The figure shows three views and two pictorial views of one solid part (mm, origin at its lowest corner). Answer the questions. A direction names the side the tool comes from. Give positions to 0.01 mm unless a question says otherwise; leave off trailing zeros. Loops run counter-clockwise (first coordinate to the right, second up) from the corner with the lowest first, then second, coordinate; pieces in that order, holes last.
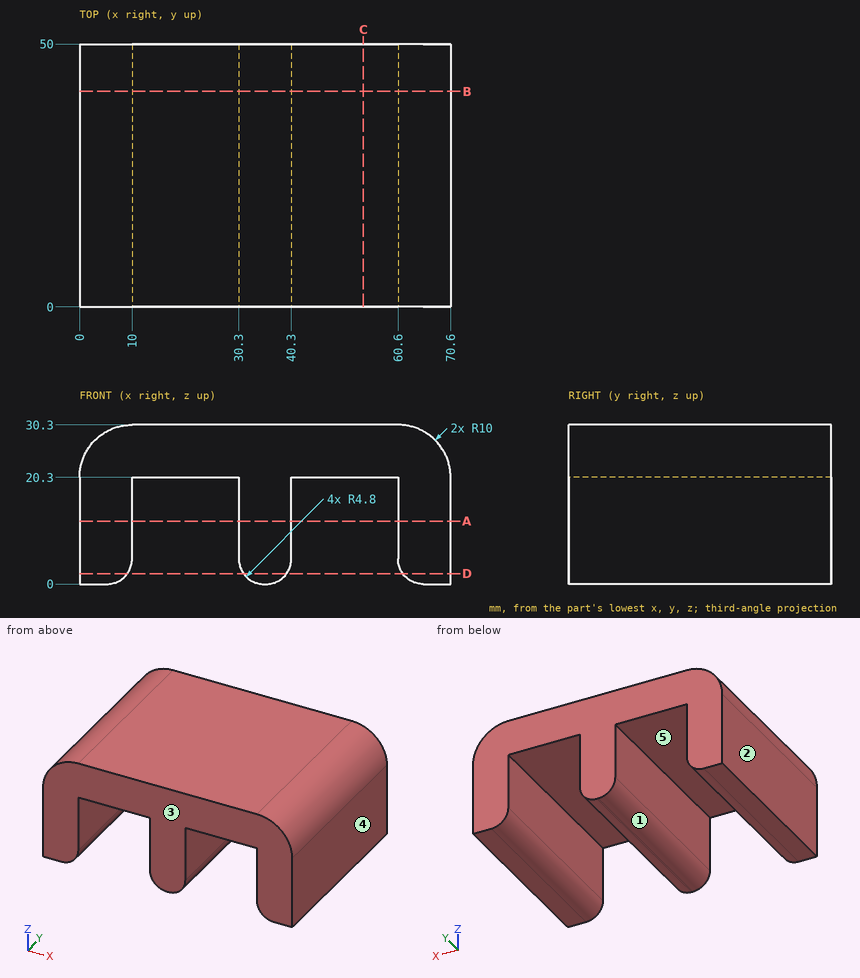
Q1. Which of the six approach directions +Z, -Z, +X, -X, +Y, -Y give full straight-line access (tool end or side, diameter ignored) to the marked faces 1 and 2?
Q2. Section A-A on z = 12 is taken. Give the vertices of the cut face in (x, y), plus the area to 3 significant figures.
Q3. Determine the mould class of the marked faces 3, 4 and 5 for opening direction X: +X half, -X half, draft (parallel to the pull), parting line (faces both ways), or undercut.
Q4. Section C-C on x = 54 is taken. Give the vertices of the cut face in (y, z).
Q5. Given pin 1 (2 mm diameter, centred on x = 62.5, y = 17, fed in from -Z); pin 2 (6 mm diameter, centred on x = 46, y = 22, fed in from -Z), each flat-ended and moving along its own axis, determine where each tip first touches the part or whether it passes through.
Q6. Section B-B on y = 41 is taken. Give the vertices of the cut face in (x, z), plus the area to 3 significant figures.
Q7. Consider line 1 along X through (y, z) = (36, 15); line 2 along X through (y, z) = (21, 2.5); line 3 along Z through (x, y) = (14, 5). Determine where each line is inside the solid, lowest interval first.
Q8. Section D-D on z = 2 is taken. Give the vertices of the cut face in (x, y).
Check result:
1. face 1: -Z, +Y, -Y
1. face 2: +Z, -Z, -X, +Y, -Y
2. outline: (0, 0) - (10, 0) - (10, 50) - (0, 50) - close; (30.3, 0) - (40.3, 0) - (40.3, 50) - (30.3, 50) - close; (60.6, 0) - (70.6, 0) - (70.6, 50) - (60.6, 50) - close
2. area: 1,500 mm2
3. face 3: draft
3. face 4: +X half
3. face 5: undercut
4. outline: (0, 20.3) - (50, 20.3) - (50, 30.3) - (0, 30.3) - close
5. pin 1: stops at z = 0.39
5. pin 2: stops at z = 20.3
6. outline: (0, 0) - (5.2, 0) arc R4.8 ccw to (10, 4.8) - (10, 20.3) - (30.3, 20.3) - (30.3, 4.8) arc R4.8 ccw to (35.1, 0) - (35.5, 0) arc R4.8 ccw to (40.3, 4.8) - (40.3, 20.3) - (60.6, 20.3) - (60.6, 4.8) arc R4.8 ccw to (65.4, 0) - (70.6, 0) - (70.6, 20.3) arc R10 ccw to (60.6, 30.3) - (10, 30.3) arc R10 ccw to (0, 20.3) - close
6. area: 1,250 mm2
7. line 1: x = 0 to 10, 30.3 to 40.3, 60.6 to 70.6
7. line 2: x = 0 to 9.41, 30.89 to 39.71, 61.19 to 70.6
7. line 3: z = 20.3 to 30.3
8. outline: (0, 0) - (9.1, 0) - (9.1, 50) - (0, 50) - close; (31.2, 0) - (39.4, 0) - (39.4, 50) - (31.2, 50) - close; (61.5, 0) - (70.6, 0) - (70.6, 50) - (61.5, 50) - close
